Work out the finished part from the listing and answer in its coordinate system (mm). A direction names the side the tool comes from. Round coordinates to 2 decimals unless told otherwise and drop trailing zeros. Order: outer loops, then holes, each group sorted by start corner. A loop starts at its lowest first (then second) coordinate and runs counter-clockwise, first axis right, second up. Notation, with made-up numbers: (84, 59.5) - (90, 59.5) arc R27 cw to (90, 90.5) - close; hole circle Ø11 at (-28, -2.75). An arc over 180 degrees is marked (long way). Put each result on its own line as item: value.
```python
from build123d import *

# Parameters (mm, degrees)
SKETCH1_R           = 3.15
BOSS_EXTRUDE1_DEPTH = 19.5
SKETCH2_R           = 0.35
BOSS_EXTRUDE2_DEPTH = 5.8
SKETCH3_R           = 6.6
BOSS_EXTRUDE3_DEPTH = 14
SKETCH4_R           = 3.4
BOSS_EXTRUDE4_DEPTH = 11
SKETCH5_R           = 1.85
CUT_EXTRUDE1_DEPTH  = 1


with BuildPart() as part:
    # Sketch1 → Boss-Extrude1 (new body)
    with BuildSketch(Plane(origin=(0, 0, 0), x_dir=(1, 0, 0), z_dir=(0, 1, 0))):
        with Locations(Location((0, 0, 0), (0, 0, 270))):
            Circle(SKETCH1_R)
    extrude(amount=BOSS_EXTRUDE1_DEPTH)

    # Sketch2 → Boss-Extrude2 (add)
    with BuildSketch(Plane.XZ):
        with Locations(Location((-1.4, 0, 0), (0, 0, 90))):
            Circle(SKETCH2_R)
        with Locations(Location((1.4, 0, 0), (0, 0, 90))):
            Circle(SKETCH2_R)
    extrude(amount=BOSS_EXTRUDE2_DEPTH)

    # Sketch3 → Boss-Extrude3 (add)
    with BuildSketch(Plane(origin=(0, 19.5, 0), x_dir=(1, 0, 0), z_dir=(0, 1, 0))):
        with Locations(Location((0, 0, 0), (0, 0, 270))):
            Circle(SKETCH3_R)
    extrude(amount=BOSS_EXTRUDE3_DEPTH)

    # Sketch4 → Boss-Extrude4 (add)
    with BuildSketch(Plane(origin=(0, 33.5, 0), x_dir=(1, 0, 0), z_dir=(0, 1, 0))):
        with Locations(Location((0, 0, 0), (0, 0, 270))):
            Circle(SKETCH4_R)
    extrude(amount=BOSS_EXTRUDE4_DEPTH)

    # Sketch5 → Cut-Extrude1 (cut)
    with BuildSketch(Plane(origin=(0, 44.5, 0), x_dir=(1, 0, 0), z_dir=(0, 1, 0))):
        with Locations(Location((0, 0, 0), (0, 0, 270))):
            Circle(SKETCH5_R)
    extrude(amount=-CUT_EXTRUDE1_DEPTH, mode=Mode.SUBTRACT)


solid = part.part
```
1) Straight lines are drawn through the part: L1, parallel to X at y = 44.3, z = 0; L2, parallel to Y at x = -4.5, z = -4.75; L3, parallel to Y at x = 0.5, z = 2. For each, find the intervals that lie inside material, in ascending order. Write a range as from..to.
Findings below:
L1: x = -3.4..-1.85, 1.85..3.4
L2: y = 19.5..33.5
L3: y = 0..44.5
2) For faces 5 (the cylindrical face through (-1.917, 9.614, -2.5)), 6 (the flat face through (-1.5, 44.5, 1.5)), determine the directions among +Z, -Z, +X, -X, +Y, -Y from which every point of the face is accessible in a straight line to the end or side of a thin tool.
Findings below:
face 5: -Y
face 6: +Z, -Z, +X, -X, +Y
3) A cutting plane is placed at A-A on x = 0. Write down the section's boundary in (y, z), then the cut area to 3 significant figures.
Findings below:
outline: (0, -3.15) - (19.5, -3.15) - (19.5, -6.6) - (33.5, -6.6) - (33.5, -3.4) - (44.5, -3.4) - (44.5, -1.85) - (43.5, -1.85) - (43.5, 1.85) - (44.5, 1.85) - (44.5, 3.4) - (33.5, 3.4) - (33.5, 6.6) - (19.5, 6.6) - (19.5, 3.15) - (0, 3.15) - close
area: 379 mm2
4) A cutting plane is placed at B-B on y = 35. Write down the section's boundary in (x, z).
Findings below:
outline: circle Ø6.8 at (0, 0)
5) A cutting plane is placed at C-C on z = 1.25. Write down the section's boundary in (x, y).
Findings below:
outline: (-6.48, 19.5) - (-2.89, 19.5) - (-2.89, 0) - (2.89, 0) - (2.89, 19.5) - (6.48, 19.5) - (6.48, 33.5) - (3.16, 33.5) - (3.16, 44.5) - (1.36, 44.5) - (1.36, 43.5) - (-1.36, 43.5) - (-1.36, 44.5) - (-3.16, 44.5) - (-3.16, 33.5) - (-6.48, 33.5) - close
6) Given pin 1 Ø4 at (x, z) = (1.5, 2.5) entering from -Y; pin 2 Ø5 at (x, y) = (0, 15) entering from +Z; pin 3 Ø3 at (x, z) = (0, 0) entering from +Y, each flat-ended and moving along its own axis, determine where each tip first touches the part or whether it passes through.
Findings below:
pin 1: stops at y = 0
pin 2: stops at z = 3.15
pin 3: stops at y = 43.5
7) A cutting plane is placed at D-D on z = -6. Write down the section's boundary in (x, y), then the cut area to 3 significant figures.
Findings below:
outline: (-2.75, 19.5) - (2.75, 19.5) - (2.75, 33.5) - (-2.75, 33.5) - close
area: 77.0 mm2
8) For a pull along Z with two mould halves and no side action, classify faces 1 (the flat face through (0, 43.5, 0)), 2 (the cylindrical face through (-1.806, 44.007, -0.401)), 3 (the cylindrical face through (-3.32, 38.92, -0.74)), 4 (the flat face through (2, 33.5, -3)) as pulls with the +Z half, pulls with the -Z half, needs draft (parallel to the pull), parting line crosses it, or undercut.
Findings below:
face 1: undercut
face 2: undercut
face 3: parting line crosses it
face 4: needs draft
